```python
from build123d import *

# Parameters (mm, degrees)
SKETCH1_W           = 120
SKETCH1_H           = 25
SKETCH1_W_2         = 110
SKETCH1_H_2         = 15
SKETCH1_W_3         = 2
SKETCH1_W_4         = 8
SKETCH1_H_3         = 2
BOSS_EXTRUDE1_DEPTH = 3


with BuildPart() as part:
    # Sketch1 → Boss-Extrude1 (new body)
    with BuildSketch(Plane(origin=(0, 0, 0), x_dir=(1, 0, 0), z_dir=(0, 1, 0))):
        with Locations((60, 12.5)):
            Rectangle(SKETCH1_W, SKETCH1_H)
        with Locations((60, 12.5)):
            Rectangle(SKETCH1_W_2, SKETCH1_H_2, mode=Mode.SUBTRACT)
        with Locations((2.5, 12.5)):
            Rectangle(SKETCH1_W_3, SKETCH1_H_2, mode=Mode.SUBTRACT)
        with Locations((117.5, 12.5)):
            Rectangle(SKETCH1_W_3, SKETCH1_H_2, mode=Mode.SUBTRACT)
        with Locations((27.787478482, 22.5)):
            Rectangle(SKETCH1_W_4, SKETCH1_H_3, mode=Mode.SUBTRACT)
    extrude(amount=BOSS_EXTRUDE1_DEPTH)


solid = part.part
```
Input: part model. Units: mm. Frame: model coordinates. A direction names the side the tool comes from. Round coordinates to 2 decimals unless told otherwise and drop trailing zeros. Order: outer loops, then holes, each group sorted by start corner. A loop starts at its lowest first (then second) coordinate and runs counter-clockwise, first axis right, second up. Notation, with made-up numbers: (-13, 36) - (17, 36) arc R11 cw to (17, 40) - close; hole circle Ø11 at (-16, 55.25). An arc over 180 degrees is marked (long way). Answer in a Markdown table with one row per item.
Item 1: Section query A-A (x = 101). Return the cut outline in (y, z).
Model answer:
| item | result |
|---|---|
| outline | (0, -25) - (3, -25) - (3, -20) - (0, -20) - close; (0, -5) - (3, -5) - (3, 0) - (0, 0) - close |
Item 2: Section query B-B (z = -17). Return the cut outline in (x, y).
Model answer:
| item | result |
|---|---|
| outline | (0, 0) - (1.5, 0) - (1.5, 3) - (0, 3) - close; (3.5, 0) - (5, 0) - (5, 3) - (3.5, 3) - close; (115, 0) - (116.5, 0) - (116.5, 3) - (115, 3) - close; (118.5, 0) - (120, 0) - (120, 3) - (118.5, 3) - close |
Item 3: Reachability of faces 1 (the flat face through (1.5, 1, -12)), 2 (the flat face through (0, 1, -12)) from +Z, -Z, +X, -X, +Y, -Y: full face, straight path, thin tool, end or side. Return the list, or none.
Model answer:
| item | result |
|---|---|
| face 1 | +Y, -Y |
| face 2 | +Z, -Z, -X, +Y, -Y |
Item 4: Section query C-C (y = 1.7). Return the cut outline in (x, z).
Model answer:
| item | result |
|---|---|
| outline | (0, -25) - (120, -25) - (120, 0) - (0, 0) - close; hole (1.5, -20) - (3.5, -20) - (3.5, -5) - (1.5, -5) - close; hole (5, -20) - (115, -20) - (115, -5) - (5, -5) - close; hole (23.79, -23.5) - (31.79, -23.5) - (31.79, -21.5) - (23.79, -21.5) - close; hole (116.5, -20) - (118.5, -20) - (118.5, -5) - (116.5, -5) - close |
Item 5: Mould query, pull axis Z, two halves, no side actions, for faces 3 (the flat face through (59, 1, -20)), 4 (the flat face through (59, 1, 0)), 5 (the flat face through (59, 0, -4)). Classes: released by +Z, released by -Z, zero draft, split by the parting line, or undercut.
Model answer:
| item | result |
|---|---|
| face 3 | undercut |
| face 4 | released by +Z |
| face 5 | zero draft |
Item 6: Line query: line 1 (X direction, y = 1.8, z = -14); line 2 (Z direction, x = 26, y = 0.2); line 3 (Z direction, x = 47.5, y = 1.3). Output: solid intervals per line, ascending.
Model answer:
| item | result |
|---|---|
| line 1 | x = 0 to 1.5, 3.5 to 5, 115 to 116.5, 118.5 to 120 |
| line 2 | z = -25 to -23.5, -21.5 to -20, -5 to 0 |
| line 3 | z = -25 to -20, -5 to 0 |
